Here's how the part is built. I have some questions about the finished solid (model axes, mm). A direction names the side the tool comes from. Round coordinates to 2 decimals unless told otherwise and drop trailing zeros. Order: outer loops, then holes, each group sorted by start corner. A loop starts at its lowest first (then second) coordinate and runs counter-clockwise, first axis right, second up. Notation, with made-up numbers: (-21.75, 35) - (-17.75, 35) arc R5 cw to (-17.75, 41) - close; hole circle Ø7 at (-23.75, 75.25). An arc over 180 degrees is marked (long way). Answer as a JSON object with one key per item and string values.
```python
from build123d import *

# Parameters (mm, degrees)
F3_D     = 5
F3_DEPTH = 8
F3_TIP   = 1.5021515476
F4_D     = 3
F5_R     = 1
F6_SIZE  = 1.5


with BuildPart() as f1:
    # F0 (on Top) → F1 (revolve)
    with BuildSketch(Plane.XY):
        with BuildLine():
            ThreePointArc((31.8614066163, 10), (12.2595141345, 16.6969251029), (0, 0))
            Line((0, 0), (82.5, 0))
            Line((82.5, 0), (82.5, 8))
            Line((82.5, 8), (61.5, 8))
            Line((61.5, 8), (60, 6.5))
            Line((60, 6.5), (54.5, 6.5))
            Line((54.5, 6.5), (54.5, 10))
            Line((54.5, 10), (31.8614066163, 10))
        make_face()
    revolve(axis=Axis((41.25, 0, 0), (1, 0, 0)))

    # F3
    with Locations(Plane.YZ.offset(82.5)):
        with Locations((0, 0)):
            Hole(F3_D / 2, depth=F3_DEPTH)
            with Locations((0, 0, -(F3_DEPTH + F3_TIP / 2))):  # 118° drill point
                Cone(0, F3_D / 2, F3_TIP, mode=Mode.SUBTRACT)

    # F4 (through all)
    with Locations(Plane.YZ.offset(82.5)):
        with Locations((0, 0)):
            Hole(F4_D / 2)

    # F5
    f5_edges = [f1.edges().sort_by_distance(p)[0] for p in [
        (54.5, -6.5, 0),
        (60, -6.5, 0),
    ]]
    fillet(f5_edges, radius=F5_R)

    # F6
    f6_edges = [f1.edges().sort_by_distance(p)[0] for p in [
        (82.5, -8, 0),
    ]]
    chamfer(f6_edges, length=F6_SIZE)


solid = f1.part
```
1. If I drill on L1, parallel to Z at x = 56, y = 0; L2, parallel to Z at x = 77, y = 0; L3, parallel to Y at x = 53.5, z = 1, over which ranges is the centre line in solid material (lowest first)? Write a range as [from, to].
Responses:
{"L1": "[-6.5, -1.5], [1.5, 6.5]", "L2": "[-8, -2.5], [2.5, 8]", "L3": "[-9.95, -1.12], [1.12, 9.95]"}
2. Thinking about a two-plate mould opening in X: for faces 4 (the face through (82, -7, 0)), 5 (the face through (57.51, 6.2, 1.95)), 6 (the face through (36.465, 0.325, -1.464)), which applies, pulls with the +X half, pulls with the -X half, needs draft (parallel to the pull), parting line crosses it, or undercut?
Responses:
{"face 4": "pulls with the +X half", "face 5": "undercut", "face 6": "needs draft"}
3. Imagine slicing it at A-A (x = 70). List the corners of the cut face in (y, z) for me, plus the area to 3 significant figures.
Responses:
{"outline": "circle Ø16 at (0, 0); hole circle Ø3 at (0, 0)", "area": "194 mm2"}
4. For P1, Ø12, axis at x = 29.5, z = -5, coming from the -Y side; P2, Ø5, axis at x = 12, z = -4, coming from the -Y side; P3, Ø12, axis at x = 37, y = 13, coming from the -Z side; P4, Ø1.5, axis at x = 57, y = 7.5, coming from the +Z side, each with a flat end and sliding along its axis, tell me the tip position at first contact or that it passes through.
Responses:
{"P1": "y = -16.04", "P2": "y = -16.96", "P3": "z = -7.14", "P4": "through"}
5. Imagine slicing it at C-C (z = 13.5). List the corners of the cut face in (x, y) for me.
Responses:
{"outline": "circle Ø22.27 at (17.5, 0)"}
6. Imagine slicing it at D-D (x = 48). List the corners of the cut face in (y, z) for me.
Responses:
{"outline": "circle Ø20 at (0, 0); hole circle Ø3 at (0, 0)"}
7. For faces 1 (the face through (82.5, -3, 0)), 2 (the face through (78.44, 0.54, -2.44)), 3 (the face through (54.5, -4, 7)), which set-ups out of +Z, -Z, +X, -X, +Y, -Y let a thin tool reach every point of the face, with its end or its side?
Responses:
{"face 1": "+Z, -Z, +X, +Y, -Y", "face 2": "+X", "face 3": "none"}
8. Imagine slicing it at B-B (y = 9). List the corners of the cut face in (x, z) for me, plus the area to 3 significant figures.
Responses:
{"outline": "(31.86, -4.36) - (54.5, -4.36) - (54.5, 4.36) - (31.86, 4.36) arc R15.01 ccw (long way) to start", "area": "901 mm2"}
